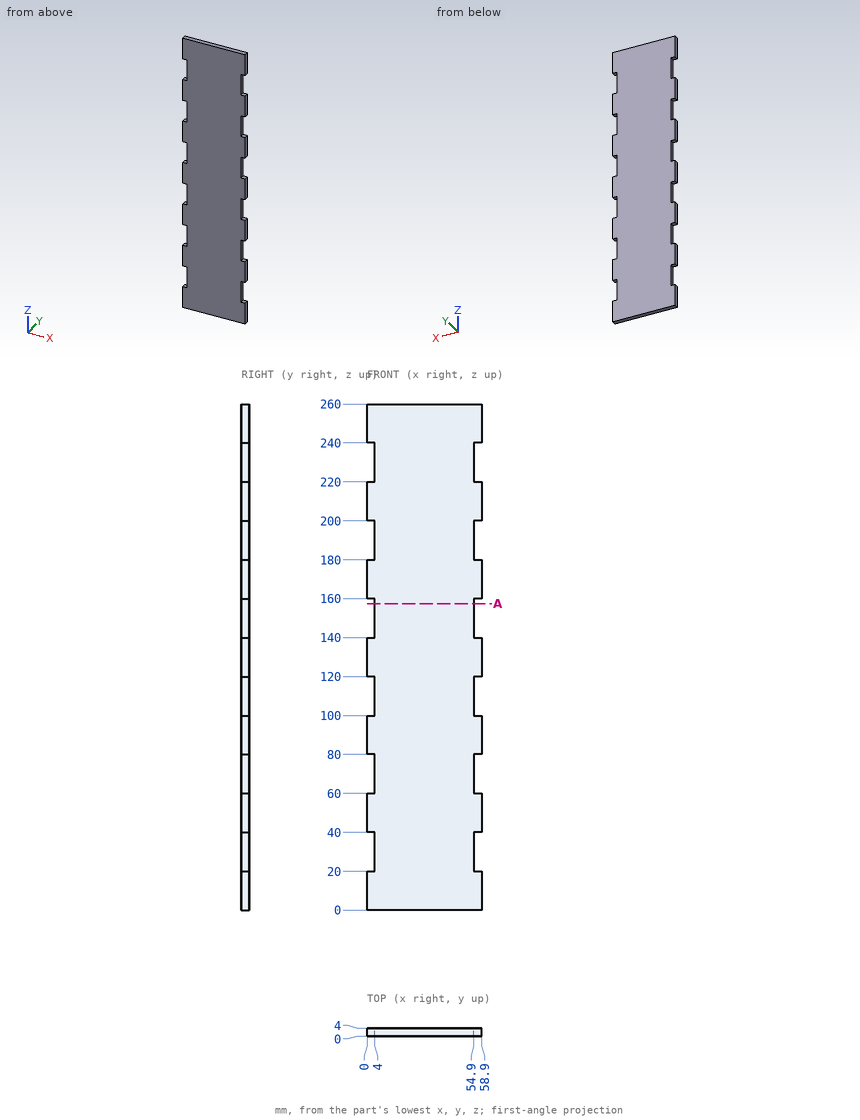
Study the drawing (mm; zero at the part's minimum x, y, z) and answer. Give positions to 0.01 mm unless a question says otherwise; leave off trailing zeros. Order: outer loops, then holes, each group sorted by start corner. A loop starts at its lowest first (then second) coordinate and runs counter-clockwise, first axis right, second up.
1) Given P1, Ø1.2, axis at x = 56.5, y = 1.5, coming from the -Z side; P2, Ø2, axis at y = 2, z = 148, coming from the -X side; P3, Ø1, axis at y = 2.5, z = 223.5, coming from the +X side, each flat-ended and moving along its own axis, determine where each tip first touches the part or whether it passes through.
Reported:
P1: stops at z = 0
P2: stops at x = 4
P3: stops at x = 54.9
2) Consider line 1 along X through (y, z) = (1.8, 236.5). Determine where the line is inside the solid, lowest interval first.
Reported:
line 1: x = 4 to 54.9
3) Find section A-A on z = 157.5. Write down the section's boundary in (x, y), then the cut area to 3 significant figures.
Reported:
outline: (4, 0) - (54.9, 0) - (54.9, 4) - (4, 4) - close
area: 204 mm2
